from build123d import *

# Parameters (mm, degrees)
SKETCH1_W               = 210
SKETCH1_H               = 90
BOSS_EXTRUDE1_DEPTH     = 3
SKETCH2_R               = 1.5
CUT_EXTRUDE1_DEPTH      = 4
SKETCH3_R               = 2
CUT_EXTRUDE2_DEPTH      = 4
CUT_EXTRUDE3_DEPTH      = 4
MIRROR3_COPY_1_SKETCH_R = 2
MIRROR3_COPY_1_DEPTH    = 4
MIRROR3_COPY_2_DEPTH    = 4
SKETCH5_R               = 3
CUT_EXTRUDE4_DEPTH      = 4


with BuildPart() as part:
    # Sketch1 → Boss-Extrude1 (new body)
    with BuildSketch(Plane(origin=(0, 0, 0), x_dir=(0, 0, -1), z_dir=(1, 0, 0))):
        Rectangle(SKETCH1_W, SKETCH1_H)
    extrude(amount=BOSS_EXTRUDE1_DEPTH)

    # Sketch2 → Cut-Extrude1 (cut, through all)
    with BuildSketch(Plane(origin=(3, 0, 0), x_dir=(0, 0, -1), z_dir=(1, 0, 0))):
        with Locations((-89, 0)):
            Circle(SKETCH2_R)
    cut_extrude1 = extrude(amount=-CUT_EXTRUDE1_DEPTH, mode=Mode.SUBTRACT)

    # Sketch3 → Cut-Extrude2 (cut, through all)
    with BuildSketch(Plane(origin=(3, 0, 0), x_dir=(0, 0, -1), z_dir=(1, 0, 0))):
        with Locations((-25, 30)):
            Circle(SKETCH3_R)
    cut_extrude2 = extrude(amount=-CUT_EXTRUDE2_DEPTH, mode=Mode.SUBTRACT)

    # Sketch4 → Cut-Extrude3 (cut, through all)
    with BuildSketch(Plane(origin=(3, 0, 0), x_dir=(0, 0, -1), z_dir=(1, 0, 0))):
        with BuildLine():
            Line((-105, 0), (-105, 45))
            Line((-105, 45), (0, 45))
            Line((0, 45), (0, 40))
            Line((0, 40), (0, 12.5))
            ThreePointArc((0, 12.5), (-5.590169944, 11.180339887), (-10, 7.5))
            Line((-10, 7.5), (-17.5, 20.490381057))
            Line((-17.5, 20.490381057), (-17.5, 30))
            ThreePointArc((-17.5, 30), (-25, 37.5), (-32.5, 30))
            Line((-32.5, 30), (-32.5, 20.490381057))
            Line((-32.5, 20.490381057), (-25, 7.5))
            Line((-25, 7.5), (-89, 7.5))
            ThreePointArc((-89, 7.5), (-94.303300859, 5.303300859), (-96.5, 0))
            Line((-96.5, 0), (-105, 0))
        make_face()
    cut_extrude3 = extrude(amount=-CUT_EXTRUDE3_DEPTH, mode=Mode.SUBTRACT)

    # Mirror2: Cut-Extrude2, Cut-Extrude3 across plane
    add(cut_extrude2.mirror(Plane.ZX), mode=Mode.SUBTRACT)
    add(cut_extrude3.mirror(Plane.ZX), mode=Mode.SUBTRACT)

    # Mirror3: Cut-Extrude3, Cut-Extrude1, Cut-Extrude2 across plane
    add(cut_extrude3.mirror(Plane.XY), mode=Mode.SUBTRACT)
    add(cut_extrude1.mirror(Plane.XY), mode=Mode.SUBTRACT)
    add(cut_extrude2.mirror(Plane.XY), mode=Mode.SUBTRACT)

    # Mirror3 copy 1 sketch → Mirror3 copy 1 (cut, through all)
    with BuildSketch(Plane(origin=(3, 0, 0), x_dir=(0, 0, 1), z_dir=(1, 0, 0))):
        with Locations((-25, 30)):
            Circle(MIRROR3_COPY_1_SKETCH_R)
    extrude(amount=-MIRROR3_COPY_1_DEPTH, mode=Mode.SUBTRACT)

    # Mirror3 copy 2 sketch → Mirror3 copy 2 (cut, through all)
    with BuildSketch(Plane(origin=(3, 0, 0), x_dir=(0, 0, 1), z_dir=(1, 0, 0))):
        with BuildLine():
            Line((-105, 0), (-105, 45))
            Line((-105, 45), (0, 45))
            Line((0, 45), (0, 40))
            Line((0, 40), (0, 12.5))
            ThreePointArc((0, 12.5), (-5.590169944, 11.180339887), (-10, 7.5))
            Line((-10, 7.5), (-17.5, 20.490381057))
            Line((-17.5, 20.490381057), (-17.5, 30))
            ThreePointArc((-17.5, 30), (-25, 37.5), (-32.5, 30))
            Line((-32.5, 30), (-32.5, 20.490381057))
            Line((-32.5, 20.490381057), (-25, 7.5))
            Line((-25, 7.5), (-89, 7.5))
            ThreePointArc((-89, 7.5), (-94.303300859, 5.303300859), (-96.5, 0))
            Line((-96.5, 0), (-105, 0))
        make_face()
    extrude(amount=-MIRROR3_COPY_2_DEPTH, mode=Mode.SUBTRACT)

    # Sketch5 → Cut-Extrude4 (cut, through all)
    with BuildSketch(Plane(origin=(3, 0, 0), x_dir=(0, 0, -1), z_dir=(1, 0, 0))):
        Circle(SKETCH5_R)
    extrude(amount=-CUT_EXTRUDE4_DEPTH, mode=Mode.SUBTRACT)


solid = part.part
The model under review builds one solid part; all positions refer to its coordinate system, in mm. A direction names the side the tool comes from. Give positions to 0.01 mm unless a question says otherwise; leave off trailing zeros. Write each loop counter-clockwise with the first axis right and the second up, starting at its lowest first coordinate (ties: lowest second). Pieces come first, ordered by that corner, then holes.
1. Draft analysis for pull direction Y (two halves, no side actions). For faces 1 (the flat face through (0, -5, 0)), 2 (the flat face through (1.521, -13.904, -13.698)), 3 (the cylindrical face through (2, 28, 25)), state which applies: +Y half, -Y half, draft (parallel to the pull), parting line (faces both ways), or undercut.
2. Add section A-A, the plane y = -14.5. Write out the cut boundary in (x, z).
3. Add section D-D, the plane z = -6. Write out the cut boundary in (x, y).
4. Wall thickness on L1, parallel to Z at x = 1.55, y = -30; L2, parallel to Z at x = 1.8, y = 26; L3, parallel to Y at x = 0.9, z = 89: over which ranges is each line inside the solid? List them lowest first.
5. Add section C-C, the plane z = 72.5. Write out the cut boundary in (x, y).
6. For P1, Ø1.5, axis at x = 1, z = 64.5, coming from the -Y side; P2, Ø1.5, axis at x = 1, z = -52.5, coming from the +Y side; P3, Ø1.5, axis at x = 0.5, y = 25.5, coming from the +Z side, all flat-tipped, find the tip position at first contact; note any pin that passes through.
7. Tool access review of faces 4 (the flat face through (1.521, 14.086, 28.802)), 5 (the flat face through (1.521, 13.904, -13.698)), 6 (the cylindrical face through (2, -28, -25)), 7 (the flat face through (1.521, -13.904, 13.698)), 8 (the flat face through (1.521, 14.086, -28.802)): name each direction out of +Z, -Z, +X, -X, +Y, -Y from which nothing blocks a thin tool from reaching the whole face with its end or side.
8. Add section B-B, the plane x = 1.8. Count the separate pieces of the cut face and the enclosed holes in it, plus the area to 3 significant figures.
Worked answers:
1. face 1: draft
1. face 2: -Y half
1. face 3: undercut
2. outline: (0, -29.04) - (3, -29.04) - (3, -14.04) - (0, -14.04) - close; (0, 14.04) - (3, 14.04) - (3, 29.04) - (0, 29.04) - close
3. outline: (0, -10.97) - (3, -10.97) - (3, 10.97) - (0, 10.97) - close
4. L1: z = -32.5 to -27, -23 to -17.5, 17.5 to 23, 27 to 32.5
4. L2: z = -32.5 to -17.5, 17.5 to 32.5
4. L3: y = -7.5 to -1.5, 1.5 to 7.5
5. outline: (0, -7.5) - (3, -7.5) - (3, 7.5) - (0, 7.5) - close
6. P1: stops at y = -7.5
6. P2: stops at y = 7.5
6. P3: stops at z = 32.5
7. face 4: +Z, +X, -X
7. face 5: +X, -X, +Y
7. face 6: +X, -X
7. face 7: +X, -X, -Y
7. face 8: -Z, +X, -X
8. separate pieces: 1
8. enclosed holes: 7
8. area: 4,600 mm2
